Source: CAD feature listing. Evaluate the final solid. Frame: model axes, mm. Face numbers are marked on the shaded views. A direction names the side the tool comes from. Round coordinates to 2 decimals unless told otherwise and drop trailing zeros. Order: outer loops, then holes, each group sorted by start corner. A loop starts at its lowest first (then second) coordinate and runs counter-clockwise, first axis right, second up. Notation, with made-up numbers: (70, 37.25) -> (85, 37.25) arc R18 cw to (85, 55.25) -> close; hole circle Ø10 at (14, 11). An arc over 180 degrees is marked (long way). Write item = value, one per line. Start each with the question number.
(1) Cut plane B-B on x = 8.75. Return the cut outline in (y, z).
(2) Ray query, line 1 (Y direction, x = -0.7, z = 0); line 2 (Y direction, x = 3, z = 0); line 3 (X direction, y = 93, z = -3.25). Return the intervals inside material, ascending.
(3) Reachability of the marked faces 3, 4 and 5 from +Z, -Z, +X, -X, +Y, -Y: full face, straight path, thin tool, end or side. Return the list, or none.
(4) Cut plane C-C on y = 36. Return the cut outline in (x, z).
(5) Cut plane D-D on z = 0. Give the number of separate pieces and of enclosed holes in the cut face, then the cut area to 3 significant figures.
(6) Contact query for flat-ended pins moving along their axis: pin 1 Ø11 at (x, y) = (0, 78) entering from +Z; pin 2 Ø2 at (x, y) = (7.5, 78) entering from +Z; pin 3 Ø10 at (x, y) = (-9.5, 56.5) entering from +Z; pin 4 Ø10 at (y, z) = (78, 6) entering from -X. Output: stop coordinate, or through.
(7) Cut plane A-A on y = 12.5. Return the cut outline in (x, z) (3 decimals).
(8) Draft query along Z for the marked faces 1 and 2. Return one class per face: released by +Z, released by -Z, zero draft, split by the parting line, or undercut.
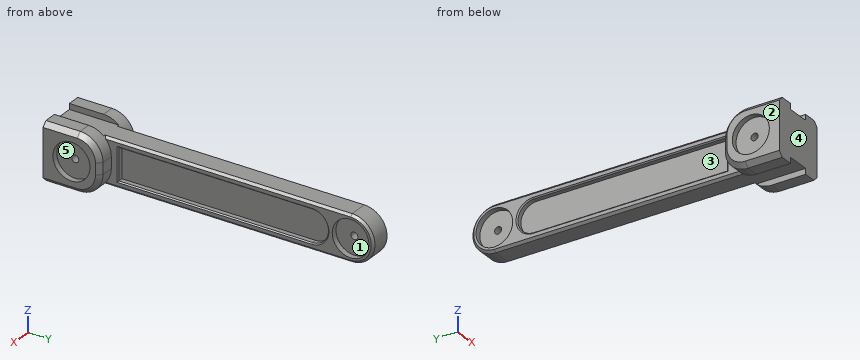
from build123d import *

# Parameters (mm, degrees)
BASE_W              = 10
BASE_H              = 20
BOSS_EXTRUDE1_DEPTH = 25
SKETCH2_R           = 8.125
SKETCH2_R_2         = 1.55
CUT_EXTRUDE1_DEPTH  = 2.5
SKETCH2_2_R         = 1.55
CUT_EXTRUDE2_DEPTH  = 38.5
BOSS_EXTRUDE2_START = 25
BASE_3_W            = 10
BASE_3_H            = 20
BOSS_EXTRUDE2_DEPTH = 115
BEARING_R           = 8.05
BEARING_R_2         = 1.55
CUT_EXTRUDE3_DEPTH  = 2.5
FILLET1_R           = 10
CHAMFER1_SIZE       = 2
CUT_EXTRUDE5_DEPTH  = 2.5
BEARING_2_R         = 1.55
CUT_EXTRUDE6_DEPTH  = 142.642154742
CHAMFER2_SIZE       = 1
CHAMFER3_SIZE       = 0.5


with BuildPart() as part:
    # Base → Boss-Extrude1 (new body)
    with BuildSketch(Plane(origin=(0, 0, 0), x_dir=(1, 0, 0), z_dir=(0, 1, 0))):
        Polygon((5, -12.5), (5, -10), (5, 10), (5, 12.5), (12.5, 12.5), (12.5, -12.5), align=None)
        Rectangle(BASE_W, BASE_H)
        Polygon((-5, 10), (-5, -10), (-5, -12.5), (-12.5, -12.5), (-12.5, 12.5), (-5, 12.5), align=None)
    extrude(amount=BOSS_EXTRUDE1_DEPTH)

    # Sketch2 → Cut-Extrude1 (cut)
    with BuildSketch(Plane.ZY.offset(12.5)):
        with Locations((0, 12.5)):
            Circle(SKETCH2_R)
        with Locations((0, 12.5)):
            Circle(SKETCH2_R_2, mode=Mode.SUBTRACT)
    cut_extrude1 = extrude(amount=-CUT_EXTRUDE1_DEPTH, mode=Mode.SUBTRACT)

    # Sketch2<2> → Cut-Extrude2 (cut, through all)
    with BuildSketch(Plane.ZY.offset(12.5)):
        with Locations((0, 12.5)):
            Circle(SKETCH2_2_R)
    extrude(amount=-CUT_EXTRUDE2_DEPTH, mode=Mode.SUBTRACT)

    # Base<3> → Boss-Extrude2 (add)
    with BuildSketch(Plane(origin=(0, 0, 0), x_dir=(1, 0, 0), z_dir=(0, 1, 0)).offset(BOSS_EXTRUDE2_START)):
        Rectangle(BASE_3_W, BASE_3_H)
    extrude(amount=BOSS_EXTRUDE2_DEPTH)

    # Mirror1: Cut-Extrude1 across plane
    add(cut_extrude1.mirror(Plane.ZY), mode=Mode.SUBTRACT)

    # Bearing → Cut-Extrude3 (cut)
    with BuildSketch(Plane.ZY.offset(5)):
        with Locations((0, 129.95)):
            Circle(BEARING_R)
        with Locations((0, 129.95)):
            Circle(BEARING_R_2, mode=Mode.SUBTRACT)
    cut_extrude3 = extrude(amount=-CUT_EXTRUDE3_DEPTH, mode=Mode.SUBTRACT)

    # Fillet1
    # the kernel refuses this fillet: 10 mm, written as the material it takes off along each edge
    with BuildSketch(Plane(origin=(37.5, 25, 12.5), x_dir=(0, -1, 0), z_dir=(-1, 0, 0)), Plane(origin=(5, 25, -12.5), x_dir=(0, -1, 0), z_dir=(1, 0, 0))) as fillet1_piece_1:
        with BuildLine():
            CenterArc((FILLET1_R, -FILLET1_R), FILLET1_R, 90, 90)
            Line((0, -FILLET1_R), (0, 0))
            Line((0, 0), (FILLET1_R, 0))
        make_face()
    extrude(amount=32.5, mode=Mode.SUBTRACT)
    with BuildSketch(Plane(origin=(37.5, 25, 12.5), x_dir=(0, -1, 0), z_dir=(-1, 0, 0))) as fillet1_piece_2_section:
        with BuildLine():
            CenterArc((FILLET1_R, -FILLET1_R), FILLET1_R, 90, 90)
            Line((0, -FILLET1_R), (0, 0))
            Line((0, 0), (FILLET1_R, 0))
        make_face()
    fillet1_piece_2 = extrude(amount=57.5, mode=Mode.PRIVATE)
    fillet1_piece_2 = split(fillet1_piece_2, bisect_by=Plane(origin=(-5, 22.736048857, 10.236048857), z_dir=(-1, 0, 0)), keep=Keep.TOP, mode=Mode.PRIVATE)
    add(fillet1_piece_2, mode=Mode.SUBTRACT)
    with BuildSketch(Plane(origin=(-20, 25, -12.5), x_dir=(0, -1, 0), z_dir=(1, 0, 0))) as fillet1_piece_3_section:
        with BuildLine():
            CenterArc((FILLET1_R, -FILLET1_R), FILLET1_R, 90, 90)
            Line((0, -FILLET1_R), (0, 0))
            Line((0, 0), (FILLET1_R, 0))
        make_face()
    fillet1_piece_3 = extrude(amount=57.5, mode=Mode.PRIVATE)
    fillet1_piece_3 = split(fillet1_piece_3, bisect_by=Plane(origin=(-5, 22.736048857, -10.236048857), z_dir=(-1, 0, 0)), keep=Keep.TOP, mode=Mode.PRIVATE)
    add(fillet1_piece_3, mode=Mode.SUBTRACT)
    with BuildSketch(Plane(origin=(-37.5, 25, -12.5), x_dir=(0, 0, 1), z_dir=(1, 0, 0)), Plane(origin=(-5, 25, 12.5), x_dir=(0, 0, -1), z_dir=(-1, 0, 0))) as fillet1_piece_4:
        with BuildLine():
            CenterArc((FILLET1_R, FILLET1_R), FILLET1_R, 180, 90)
            Line((0, FILLET1_R), (0, 0))
            Line((0, 0), (FILLET1_R, 0))
        make_face()
    extrude(amount=32.5, mode=Mode.SUBTRACT)
    with BuildSketch(Plane(origin=(-37.5, 25, -12.5), x_dir=(0, 0, 1), z_dir=(1, 0, 0))) as fillet1_piece_5_section:
        with BuildLine():
            CenterArc((FILLET1_R, FILLET1_R), FILLET1_R, 180, 90)
            Line((0, FILLET1_R), (0, 0))
            Line((0, 0), (FILLET1_R, 0))
        make_face()
    fillet1_piece_5 = extrude(amount=57.5, mode=Mode.PRIVATE)
    fillet1_piece_5 = split(fillet1_piece_5, bisect_by=Plane(origin=(5, 22.736048857, -10.236048857), z_dir=(1, 0, 0)), keep=Keep.TOP, mode=Mode.PRIVATE)
    add(fillet1_piece_5, mode=Mode.SUBTRACT)
    with BuildSketch(Plane(origin=(20, 25, 12.5), x_dir=(0, 0, -1), z_dir=(-1, 0, 0))) as fillet1_piece_6_section:
        with BuildLine():
            CenterArc((FILLET1_R, FILLET1_R), FILLET1_R, 180, 90)
            Line((0, FILLET1_R), (0, 0))
            Line((0, 0), (FILLET1_R, 0))
        make_face()
    fillet1_piece_6 = extrude(amount=57.5, mode=Mode.PRIVATE)
    fillet1_piece_6 = split(fillet1_piece_6, bisect_by=Plane(origin=(5, 22.736048857, 10.236048857), z_dir=(1, 0, 0)), keep=Keep.TOP, mode=Mode.PRIVATE)
    add(fillet1_piece_6, mode=Mode.SUBTRACT)
    with BuildSketch(Plane(origin=(30, 140, 10), x_dir=(0, -1, 0), z_dir=(-1, 0, 0)), Plane(origin=(-30, 140, -10), x_dir=(0, -1, 0), z_dir=(1, 0, 0))) as fillet1_piece_7:
        with BuildLine():
            CenterArc((FILLET1_R, -FILLET1_R), FILLET1_R, 90, 90)
            Line((0, -FILLET1_R), (0, 0))
            Line((0, 0), (FILLET1_R, 0))
        make_face()
    extrude(amount=60, mode=Mode.SUBTRACT)

    # Chamfer1
    chamfer1_edges = [part.edges().sort_by_distance(p)[0] for p in [
        (12.5, 7.5, -12.5),
        (12.5, 25, 0),
        (12.5, 7.5, 12.5),
        (12.5, 22.071067812, 9.571067812),
        (12.5, 22.071067812, -9.571067812),
        (-12.5, 25, 0),
        (-12.5, 7.5, 12.5),
        (-12.5, 7.5, -12.5),
        (-12.5, 22.071067812, 9.571067812),
        (-12.5, 22.071067812, -9.571067812),
    ]]
    chamfer(chamfer1_edges, length=CHAMFER1_SIZE)

    # Sketch4 → Cut-Extrude5 (cut)
    with BuildSketch(Plane(origin=(5, 0, 0), x_dir=(0, 0, -1), z_dir=(1, 0, 0))):
        with BuildLine():
            Line((-7, 28), (7, 28))
            Line((7, 28), (7, 112.95))
            ThreePointArc((7, 112.95), (0, 119.95), (-7, 112.95))
            Line((-7, 112.95), (-7, 28))
        make_face()
    cut_extrude5 = extrude(amount=-CUT_EXTRUDE5_DEPTH, mode=Mode.SUBTRACT)

    # Mirror2: Cut-Extrude3, Cut-Extrude5 across plane
    add(cut_extrude3.mirror(Plane.ZY), mode=Mode.SUBTRACT)
    add(cut_extrude5.mirror(Plane.ZY), mode=Mode.SUBTRACT)

    # Bearing<2> → Cut-Extrude6 (cut, through all)
    with BuildSketch(Plane.ZY.offset(5)):
        with Locations((0, 129.95)):
            Circle(BEARING_2_R)
    extrude(amount=-CUT_EXTRUDE6_DEPTH, mode=Mode.SUBTRACT)

    # Chamfer2
    chamfer2_edges = [part.edges().sort_by_distance(p)[0] for p in [
        (5, 140, 0),
        (5, 140, 0),
        (5, 75.807189139, 10),
        (-5, 75.807189139, 10),
        (-5, 75.807189139, -10),
        (5, 75.807189139, -10),
        (-5, 140, 0),
        (-5, 140, 0),
    ]]
    chamfer(chamfer2_edges, length=CHAMFER2_SIZE)

    # Chamfer3
    chamfer3_edges = [part.edges().sort_by_distance(p)[0] for p in [
        (5, 119.95, 0),
        (5, 70.475, 7),
        (5, 28, 0),
        (5, 70.475, -7),
        (-5, 119.95, 0),
        (-5, 70.475, 7),
        (-5, 28, 0),
        (-5, 70.475, -7),
    ]]
    chamfer(chamfer3_edges, length=CHAMFER3_SIZE)


solid = part.part
Evaluation:
q1.outline = (0, -12.5) -> (15, -12.5) arc R10 ccw to (25, -2.5) -> (25, 2.5) arc R10 ccw to (15, 12.5) -> (0, 12.5) -> close; hole circle Ø3.1 at (12.5, 0)
q2.line_1 = 0 to 10.95, 14.05 to 128.4, 131.5 to 140
q2.line_2 = 0 to 10.95, 14.05 to 28, 119.95 to 121.9, 138 to 140
q2.line_3 = -2.5 to 2.5
q3.face_3 = -X
q3.face_4 = +Z, -Z, +X, -X, -Y
q3.face_5 = +X
q4.outline = (-5, -9) -> (-4, -10) -> (4, -10) -> (5, -9) -> (5, -7.5) -> (4.5, -7) -> (2.5, -7) -> (2.5, 7) -> (4.5, 7) -> (5, 7.5) -> (5, 9) -> (4, 10) -> (-4, 10) -> (-5, 9) -> (-5, 7.5) -> (-4.5, 7) -> (-2.5, 7) -> (-2.5, -7) -> (-4.5, -7) -> (-5, -7.5) -> close
q5.separate_pieces = 3
q5.enclosed_holes = 0
q5.area = 1,070 mm^2
q6.pin_1 = 10
q6.pin_2 = through
q6.pin_3 = 9.5
q6.pin_4 = -5
q7.outline = (-12.5, -10.5) -> (-10.5, -12.5) -> (-5, -12.5) -> (-5, -10) -> (5, -10) -> (5, -12.5) -> (10.5, -12.5) -> (12.5, -10.5) -> (12.5, -8.125) -> (10, -8.125) -> (10, -1.55) -> (-10, -1.55) -> (-10, -8.125) -> (-12.5, -8.125) -> close; (-12.5, 8.125) -> (-10, 8.125) -> (-10, 1.55) -> (10, 1.55) -> (10, 8.125) -> (12.5, 8.125) -> (12.5, 10.5) -> (10.5, 12.5) -> (5, 12.5) -> (5, 10) -> (-5, 10) -> (-5, 12.5) -> (-10.5, 12.5) -> (-12.5, 10.5) -> close
q8.face_1 = undercut
q8.face_2 = zero draft
